Read the model definition and answer for the solid it produces. Units are mm, in the model's axes. A direction names the side the tool comes from. Give positions to 0.01 mm unless a question says otherwise; leave off trailing zeros. Loops run counter-clockwise (first coordinate to the right, second up) from the corner with the lowest first, then second, coordinate; pieces in that order, holes last.
(1) Find section D-D, the plane x = -455. Write down the section's boundary in (y, z), then the cut area to 3 significant figures.
(2) Which of the six approach directions +Z, -Z, +X, -X, +Y, -Y give full straight-line access (tool end or side, diameter ignored) to faces 4 (the face through (-463, 3, 92.18)), 5 (the face through (-436, 3, 106.18)), 6 (the face through (-459.438, 3, 91))?
(3) Find section C-C, the plane z = 93.25. Write down the section's boundary in (x, y), then the cut area to 3 significant figures.
(4) Find section A-A, the plane z = 108. Write down the section's boundary in (x, y).
(5) Find section B-B, the plane x = -436. Write down the section's boundary in (y, z), then the cut area to 3 significant figures.
(6) Straight lines are drawn through the part: probe 1 along X at (y, z) = (4.65, 111.5); probe 2 along Z at (x, y) = (-459.5, 1.2); probe 3 along Z at (x, y) = (-451, 3.4). For each, find the intervals that lie inside material, in ascending order.
(7) Determine the mould class of faces 1 (the face through (-455.538, 3, 111)), 2 (the face through (-430, 3, 113.18)), 3 (the face through (-465.438, 3, 104)) for opening direction X: pulls with the +X half, pulls with the -X half, needs draft (parallel to the pull), parting line crosses it, or undercut.
(8) Each of these flat-tipped pins is pushed along its axis until it touches: P1, Ø1.1, axis at y = 2, z = 96, coming from the +X side; P2, Ø0.7, axis at y = 3.5, z = 91.5, coming from the +X side; P3, Ø5.5, axis at x = -435.31, z = 94.18, coming from the +Y side; P4, Ø0.9, axis at y = 2, z = 93.5, coming from the -X side. Where does it stop, or does it pass through?
```python
from build123d import *

# Parameters (mm, degrees)
DODANIE_WYCI_GNI_CIE1_DEPTH = 6
WYTNIJ_WYCI_GNI_CIE1_DEPTH  = 6
SZYK_LINIOWY1_COUNT         = 2
SZYK_LINIOWY1_PITCH         = 18
WYTNIJ_WYCI_GNI_CIE2_DEPTH  = 6
SZKIC6_R                    = 1.75
SZKIC6_R_2                  = 1.55
WYTNIJ_WYCI_GNI_CIE3_DEPTH  = 6


with BuildPart() as part:
    # Szkic3 → Dodanie-wyciągnięcie1 (new body)
    with BuildSketch(Plane(origin=(0, 0, 0), x_dir=(1, 0, 0), z_dir=(0, 1, 0))):
        with BuildLine():
            Line((-425.43845817, -113.179624371), (-425.43845817, -103.179624371))
            ThreePointArc((-425.43845817, -103.179624371), (-431.296322547, -89.037488748), (-445.43845817, -83.179624371))
            Line((-445.43845817, -83.179624371), (-465.43845817, -83.179624371))
            Line((-465.43845817, -83.179624371), (-465.43845817, -113.179624371))
            Line((-465.43845817, -113.179624371), (-425.43845817, -113.179624371))
        make_face()
    extrude(amount=DODANIE_WYCI_GNI_CIE1_DEPTH)

    # Szkic4 → Wytnij-wyciągnięcie1 (cut)
    with BuildSketch(Plane(origin=(0, 6, 0), x_dir=(1, 0, 0), z_dir=(0, 1, 0))):
        Polygon((-434.43845817, -113.179624371), (-437.53845817, -113.179624371), (-437.53845817, -109.179624371), (-438.91345817, -109.179624371), (-438.91345817, -107.179624371), (-437.53845817, -107.179624371), (-437.53845817, -106.179624371), (-434.43845817, -106.179624371), (-434.43845817, -107.179624371), (-433.06345817, -107.179624371), (-433.06345817, -109.179624371), (-434.43845817, -109.179624371), align=None)
    wytnij_wyci_gni_cie1 = extrude(amount=-WYTNIJ_WYCI_GNI_CIE1_DEPTH, mode=Mode.SUBTRACT)

    # Szyk liniowy1: Wytnij-wyciągnięcie1 ×2
    with Locations(*[(-i * SZYK_LINIOWY1_PITCH, 0, 0) for i in range(1, SZYK_LINIOWY1_COUNT)]):
        add(wytnij_wyci_gni_cie1, mode=Mode.SUBTRACT)

    # Szkic5 → Wytnij-wyciągnięcie2 (cut)
    with BuildSketch(Plane(origin=(0, 6, 0), x_dir=(1, 0, 0), z_dir=(0, 1, 0))):
        Polygon((-465.43845817, -95.279624371), (-465.43845817, -92.179624371), (-461.43845817, -92.179624371), (-461.43845817, -90.804624371), (-459.43845817, -90.804624371), (-459.43845817, -92.179624371), (-458.43845817, -92.179624371), (-458.43845817, -95.279624371), (-459.43845817, -95.279624371), (-459.43845817, -96.654624371), (-461.43845817, -96.654624371), (-461.43845817, -95.279624371), align=None)
    extrude(amount=-WYTNIJ_WYCI_GNI_CIE2_DEPTH, mode=Mode.SUBTRACT)

    # Szkic6 → Wytnij-wyciągnięcie3 (cut)
    with BuildSketch(Plane(origin=(0, 6, 0), x_dir=(1, 0, 0), z_dir=(0, 1, 0))):
        with Locations(Location((-435.310416703, -94.179624371, 0), (0, 0, 270))):
            Circle(SZKIC6_R)
        with Locations(Location((-450.310416703, -94.179624371, 0), (0, 0, 270))):
            Circle(SZKIC6_R_2)
    extrude(amount=-WYTNIJ_WYCI_GNI_CIE3_DEPTH, mode=Mode.SUBTRACT)


solid = part.part
```
Entries:
1. outline: (0, 83.18) - (6, 83.18) - (6, 106.18) - (0, 106.18) - close
1. area: 138 mm2
2. face 4: -X, +Y, -Y
2. face 5: +Z, +Y, -Y
2. face 6: +Y, -Y
3. outline: (-458.44, 0) - (-451.55, 0) - (-451.55, 6) - (-458.44, 6) - close; (-449.07, 0) - (-436.79, 0) - (-436.79, 6) - (-449.07, 6) - close; (-433.83, 0) - (-428.08, 0) - (-428.08, 6) - (-433.83, 6) - close
3. area: 149 mm2
4. outline: (-465.44, 0) - (-456.91, 0) - (-456.91, 6) - (-465.44, 6) - close; (-451.06, 0) - (-438.91, 0) - (-438.91, 6) - (-451.06, 6) - close; (-433.06, 0) - (-425.44, 0) - (-425.44, 6) - (-433.06, 6) - close
5. outline: (0, 85.55) - (6, 85.55) - (6, 92.57) - (0, 92.57) - close; (0, 95.79) - (6, 95.79) - (6, 106.18) - (0, 106.18) - close
5. area: 104 mm2
6. probe 1: x = -465.44 to -455.54, -452.44 to -437.54, -434.44 to -425.44
6. probe 2: z = 83.18 to 90.8, 96.65 to 113.18
6. probe 3: z = 83.18 to 92.79, 95.57 to 113.18
7. face 1: undercut
7. face 2: needs draft
7. face 3: pulls with the -X half
8. P1: stops at x = -426.57
8. P2: stops at x = -428.96
8. P3: stops at y = 6
8. P4: stops at x = -458.44
